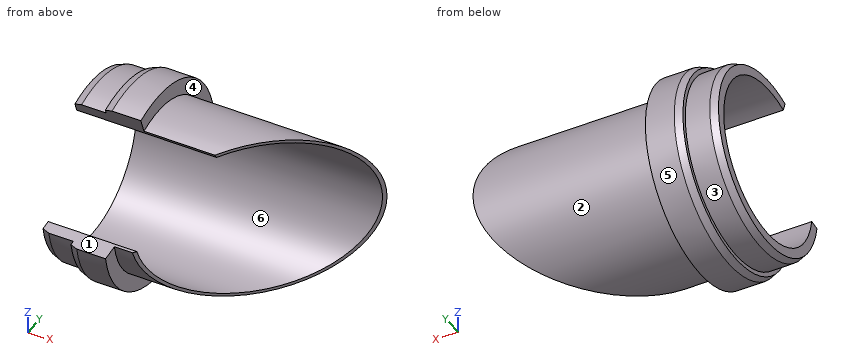
from build123d import *
from OCP.BRepFilletAPI import BRepFilletAPI_MakeChamfer

# Parameters (mm, degrees)
CUT_EXTRUDE1_DEPTH      = 198.818204546
CUT_EXTRUDE1_DEPTH_BACK = 198.818204546
CHAMFER1_SIZE           = 5
CHAMFER1_SIZE2          = 1.819851171
CUT_EXTRUDE3_DEPTH      = 198.818204546
CUT_EXTRUDE3_DEPTH_BACK = 198.818204546


with BuildPart() as part:
    # Sketch1 → Revolve1 (revolve)
    with BuildSketch(Plane.XY, mode=Mode.PRIVATE) as revolve1_sk:
        Polygon((170.74, 55.05), (172.74, 57.05), (47, 57.05), (47, 68.165), (22, 68.165), (22, 63.4), (0, 63.4), (0, 55.05), align=None)
        Polygon((172.74, 55.05), (172.74, 57.05), (170.74, 55.05), align=None)
    revolve(revolve1_sk.sketch.rotate(Axis((0, 0, 0), (1, 0, 0)), 90), axis=Axis((0, 0, 0), (1, 0, 0)))

    # Sketch1_3 → Cut-Extrude1 (cut, two sides: drawn at the far end of the back side and taken through both)
    with BuildSketch(Plane.XY.offset(-CUT_EXTRUDE1_DEPTH_BACK)):
        Polygon((182.74, 67.05), (172.74, 57.05), (172.74, 55.05), (170.74, 55.05), (-17.26, -132.95), (182.74, -132.95), align=None)
        Polygon((172.74, 55.05), (172.74, 57.05), (170.74, 55.05), align=None)
    extrude(amount=CUT_EXTRUDE1_DEPTH + CUT_EXTRUDE1_DEPTH_BACK, mode=Mode.SUBTRACT)

    # Chamfer1: one chamfer whose edges measure the first distance from different faces: ONE call of the kernel's chamfer builder (chamfer() names one face for all edges)
    chamfer1_edges_1 = [part.edges().sort_by_distance(p)[0] for p in [
        (0, 0, -63.4),
    ]]
    chamfer1_side_1 = [part.faces().sort_by_distance(p)[0] for p in [
        (11, 0, -63.4),
    ]]
    chamfer1_edges_2 = [part.edges().sort_by_distance(p)[0] for p in [
        (22, 0, -68.165),
    ]]
    chamfer1_side_2 = [part.faces().sort_by_distance(p)[0] for p in [
        (34.5, 0, -68.165),
    ]]
    chamfer1 = BRepFilletAPI_MakeChamfer(part.part.solid().wrapped)
    for e in chamfer1_edges_1:
        chamfer1.Add(CHAMFER1_SIZE, CHAMFER1_SIZE2, e.wrapped, chamfer1_side_1[0].wrapped)  # the first distance lies on this face
    for e in chamfer1_edges_2:
        chamfer1.Add(CHAMFER1_SIZE, CHAMFER1_SIZE2, e.wrapped, chamfer1_side_2[0].wrapped)  # the first distance lies on this face
    add(Compound.cast(chamfer1.Shape()), mode=Mode.REPLACE)

    # Sketch2 → Cut-Extrude3 (cut, two sides: drawn at the far end of the back side and taken through both)
    with BuildSketch(Plane(origin=(0, 0, 0), x_dir=(0, 0, -1), z_dir=(1, 0, 0)).offset(-CUT_EXTRUDE3_DEPTH_BACK)):
        Polygon((0, 0), (-302.22251614, -110), (19.395967878, -110), align=None)
    extrude(amount=CUT_EXTRUDE3_DEPTH + CUT_EXTRUDE3_DEPTH_BACK, mode=Mode.SUBTRACT)


solid = part.part
Verification items for the finished model (mm, model axes). Face numbers are marked on the shaded views. A direction names the side the tool comes from. Round coordinates to 2 decimals unless told otherwise and drop trailing zeros. Loops run counter-clockwise (first coordinate to the right, second up) from the corner with the lowest first, then second, coordinate; pieces in that order, holes last. Notation, with made-up numbers: (81.5, 35) - (117.5, 35) arc R28 cw to (117.5, 71) - close; hole circle Ø6 at (24.25, 44.25). An arc over 180 degrees is marked (long way). Use a Markdown table: item, result. Add a question column.
1. Section check C-C, the plane x = 138. Record the boundary of the cut face in (y, z), plus the area to 3 significant figures.
2. Access from +Z, -Z, +X, -X, +Y, -Y to the whole of each face (thin tool, end or side, straight path). Record for the marked faces 1, 2 and 3.
3. Release check for a two-part mould opening along Z. For the marked faces 4, 5 and 6 record: released by +Z, released by -Z, zero draft, split by the parting line, or undercut.
4. Section check B-B, the plane z = 0. Record the boundary of the cut face in (x, y) (3 decimals), plus the area to 3 significant figures.
5. Section check A-A, the plane y = 0. Record the boundary of the cut face in (x, z) (3 decimals), plus the area to 3 significant figures.
6. Thickness scan on probe 1 along Z at (x, y) = (85, 0); probe 2 along Y at (x, z) = (102, 0); probe 3 along X at (y, z) = (54.5, 33). Record the ranges inside material, lowest first. Write a range as [from, to].
7. Section check D-D, the plane x = 32. Record the boundary of the cut face in (y, z) (3 decimals).
8. Gauge pin test, flat ends, axial feed: pin 1 (10 mm diameter, centred on x = 29, z = 13, fed in from +Y); pin 2 (1 mm diameter, centred on x = 40, z = -24.5, fed in from -Y); pin 3 (4 mm diameter, centred on x = 45, z = -46.5, fed in from +Y); pin 4 (4 mm diameter, centred on y = 23, z = 48.5, fed in from -X). Record the tip position at first contact, or that the pin passes through.
Checks:
| question | item | result |
|---|---|---|
| 1 | outline | (22.31, -52.51) arc R57.05 ccw to (22.31, 52.51) - (22.31, 50.33) arc R55.05 cw to (22.31, -50.33) - close |
| 1 | area | 260 mm^2 |
| 2 | face 1 | +Z, +X, -X, -Y |
| 2 | face 2 | +X |
| 2 | face 3 | -X |
| 3 | face 4 | zero draft |
| 3 | face 5 | split by the parting line |
| 3 | face 6 | undercut |
| 4 | outline | (0, 55.05) - (170.74, 55.05) - (172.74, 57.05) - (47, 57.05) - (47, 68.165) - (27, 68.165) - (22, 66.345) - (22, 63.4) - (5, 63.4) - (0, 61.58) - close |
| 4 | area | 752 mm^2 |
| 5 | outline | (0, -61.58) - (5, -63.4) - (22, -63.4) - (22, -66.345) - (27, -68.165) - (47, -68.165) - (47, -57.05) - (115.69, -57.05) - (115.69, -55.05) - (0, -55.05) - close; (0, 55.05) - (115.69, 55.05) - (115.69, 57.05) - (47, 57.05) - (47, 68.165) - (27, 68.165) - (22, 66.345) - (22, 63.4) - (5, 63.4) - (0, 61.58) - close |
| 5 | area | 1,280 mm^2 |
| 6 | probe 1 | z = [-57.05, -55.05], [55.05, 57.05] |
| 6 | probe 2 | y = [55.05, 57.05] |
| 6 | probe 3 | x = [22, 47] |
| 7 | outline | (-67.129, -11.837) arc R68.165 ccw (long way) to (-23.314, 64.054) - (-18.828, 51.73) arc R55.05 cw (long way) to (-54.214, -9.559) - close |
| 8 | pin 1 | stops at y = 67.69 |
| 8 | pin 2 | stops at y = -63.8 |
| 8 | pin 3 | stops at y = 51.64 |
| 8 | pin 4 | stops at x = 0 |
